from build123d import *

# Parameters (mm, degrees)
F4_W          = 126.554620702
F4_H          = 16.890758596
F5_DEPTH      = 25
F5_DEPTH_BACK = 25
F6_W          = 22.8272504394
F6_H          = 2


# Not quite as in the source:
# - a pattern or mirror of a feature is missing from the dataset's text; its kind, count and spacing are read off the source's solid


with BuildPart() as f1:
    # F0 (on Front) → F1 (revolve)
    with BuildSketch(Plane.XZ):
        with BuildLine():
            Line((0, 50), (0, -50))
            ThreePointArc((0, -50), (50, 0), (0, 50))
        make_face()
    revolve(axis=Axis((0, 0, 0), (0, 0, -1)))

    # F2 (on Right) → F3 (revolve, cut)
    with BuildSketch(Plane.YZ):
        with BuildLine():
            Line((-55, 52.4620511452), (-56.5292847679, 7.5011055772))
            ThreePointArc((-56.5292847679, 7.5011055772), (-33.8192423865, 29.2351357427), (-55, 52.4620511452))
        make_face()
    revolve(axis=Axis((0, -55.7646423839, 29.9815783612), (0, -0.033993967, -0.9994220381)), mode=Mode.SUBTRACT)

    # F4 (on Front) → F5 (cut, two sides)
    with BuildSketch(Plane.XZ) as f5_sk:
        with Locations((-0.5138665438, 53.445379298)):
            Rectangle(F4_W, F4_H)
    f5 = extrude(amount=-F5_DEPTH, mode=Mode.SUBTRACT) + extrude(f5_sk.sketch, amount=F5_DEPTH_BACK, mode=Mode.SUBTRACT)

    # F5_copies: F5 across plane
    add(f5.mirror(Plane(origin=(0, 0, 0), x_dir=(-1, 0, 0), z_dir=(0, 0, -1))), mode=Mode.SUBTRACT)

    # F6 (on Front) → F7 (revolve, cut)
    with BuildSketch(Plane.XZ):
        with Locations((-59.4136252197, 0)):
            Rectangle(F6_W, F6_H)
    revolve(axis=Axis((0, 0, 0), (0, 0, -1)), mode=Mode.SUBTRACT)


solid = f1.part
Input: part model. Units: mm. Frame: model coordinates. Give positions to 0.01 mm unless a question says otherwise; leave off trailing zeros. Write each loop counter-clockwise with the first axis right and the second up, starting at its lowest first coordinate (ties: lowest second). Pieces come first, ordered by that corner, then holes. Notation, with made-up numbers: (-38.5, 52) -> (-33.5, 52) arc R21 cw to (-33.5, 67) -> close; hole circle Ø7 at (29, 48). An arc over 180 degrees is marked (long way). Use one line per item in the form item = value. Start each with the question number.
1) Section query C-C on z = -35. Return the cut outline in (x, y).
2) Draft query along Z for faces 1 (the flat face through (19, 45, -1)), 2 (the flat face through (0, 0, 45)), 3 (the flat face through (0, 0, -45)). Return one class per face: pulls with the +Z half, pulls with the -Z half, needs draft (parallel to the pull), parting line crosses it, or undercut.
3) Pin query (flat end, axial travel): pin 1 (4 mm diameter, centred on x = 14, y = -23, fed in from +Z); pin 2 (8 mm diameter, centred on y = 24, z = -1.5, fed in from -X); pin 3 (3 mm diameter, centred on x = 28, y = -20.5, fed in from -Z). Return the tip coordinate at first contact, or that it passes through.
4) Section query B-B on y = 0. Return the cut outline in (x, z).
5) Ray query, probe 1 along Z at (x, y) = (-6, -21); probe 2 along X at (y, z) = (-37.5, 25); probe 3 along Z at (x, y) = (28.5, 23.5). Return the intervals inside material, ascending. Write a range as from..to.
Outcome:
q1.outline = circle Ø71.41 at (0, 0)
q2.face_1 = undercut
q2.face_2 = pulls with the +Z half
q2.face_3 = pulls with the -Z half
q3.pin_1 = 43.34
q3.pin_2 = -45.81
q3.pin_3 = -37.38
q4.outline = (-49.99, -1) arc R50 ccw to (-21.79, -45) -> (21.79, -45) arc R50 ccw to (49.99, -1) -> (48, -1) -> (48, 1) -> (49.99, 1) arc R50 ccw to (21.79, 45) -> (-21.79, 45) arc R50 ccw to (-49.99, 1) -> (-48, 1) -> (-48, -1) -> close
q5.probe_1 = -44.98..44.98
q5.probe_2 = -21.65..-11.14, 11.14..21.65
q5.probe_3 = -33.7..33.7
